The listing builds one solid part. Answer for the finished solid, in the listing's coordinates (mm). Face numbers are marked on the shaded views. A direction names the side the tool comes from. Give positions to 0.01 mm unless a question says otherwise; leave off trailing zeros. Loops run counter-clockwise (first coordinate to the right, second up) from the corner with the lowest first, then second, coordinate; pieces in that order, holes last. Notation, with made-up numbers: (56.25, 37.25) - (86.25, 37.25) arc R11 ccw to (86.25, 47.25) - close; hole circle Ø7 at (41.25, 5.25). An arc over 180 degrees is marked (long way). Write each question's results on one line, items separated by ' | '.
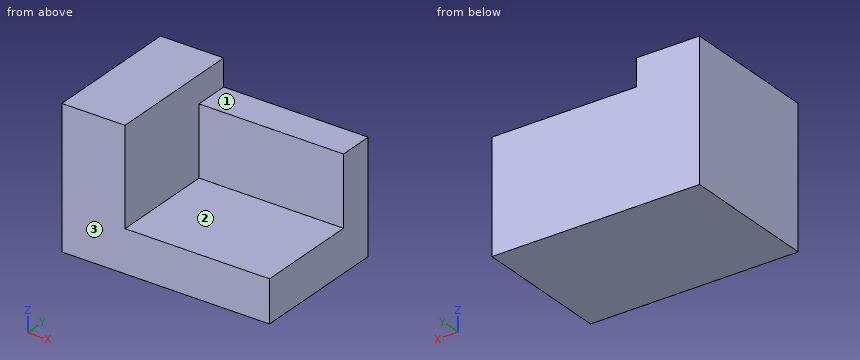
from build123d import *

# Parameters (mm, degrees)
F1_DEPTH = 25.4
F2_W     = 6.35
F2_H     = 12.7
F3_DEPTH = 26.509916


with BuildPart() as f1:
    # F0 (on Front) → F1 (new body)
    with BuildSketch(Plane.XZ):
        Polygon((0, 25.4), (0, 0), (38.1, 0), (38.1, 7.726722), (11.590084, 7.726722), (11.590084, 25.4), align=None)
    extrude(amount=F1_DEPTH)

    # F2 (on face) → F3 (join, through all)
    with BuildSketch(Plane.YZ.offset(11.590084)):
        with Locations((-3.175, 14.076722)):
            Rectangle(F2_W, F2_H)
    extrude(amount=F3_DEPTH)


solid = f1.part
Item 1: Find the intervals of material crossed by line 1 along Y through (x, z) = (15, 14); line 2 along X through (y, z) = (-18.25, 20.75); line 3 along Z through (x, y) = (12.5, -17.25), in increasing order. Write a range as [from, to].
Values found:
line 1: y = [-6.35, 0] | line 2: x = [0, 11.59] | line 3: z = [0, 7.73]
Item 2: For the marked faces 1, 2 and 3, determine the directions among +Z, -Z, +X, -X, +Y, -Y from which every point of the face is accessible in a straight line to the end or side of a thin tool.
Values found:
face 1: +Z, +X, +Y, -Y | face 2: +Z, +X, -Y | face 3: +Z, -Z, +X, -X, -Y
Item 3: A cutting plane is placed at A-A, the plane x = 35. Determine the outline of the cut face in (y, z), plus the area to 3 significant figures.
Values found:
outline: (-25.4, 0) - (0, 0) - (0, 20.43) - (-6.35, 20.43) - (-6.35, 7.73) - (-25.4, 7.73) - close | area: 277 mm²
Item 4: Flat-ended cylindrical pins translate along their axes: P1, Ø3, axis at x = 26, y = -17.5, coming from the +Z side; P2, Ø1, axis at y = -13.5, z = 19, coming from the +X side; P3, Ø15, axis at x = 21, y = -12.5, coming from the +Z side. Find the tip coordinate at first contact, or state that the pin passes through.
Values found:
P1: stops at z = 7.73 | P2: stops at x = 11.59 | P3: stops at z = 20.43
Item 5: A cutting plane is placed at B-B, the plane z = 12.25. Determine the outline of the cut face in (x, y), plus the area to 3 significant figures.
Values found:
outline: (0, -25.4) - (11.59, -25.4) - (11.59, -6.35) - (38.1, -6.35) - (38.1, 0) - (0, 0) - close | area: 463 mm²
Item 6: A cutting plane is placed at C-C, the plane z = 21.75. Determine the outline of the cut face in (x, y), plus the area to 3 significant figures.
Values found:
outline: (0, -25.4) - (11.59, -25.4) - (11.59, 0) - (0, 0) - close | area: 294 mm²
